```python
from build123d import *

# Parameters (mm, degrees)
SKETCH3_R           = 5.25
SKETCH3_R_2         = 21
BOSS_EXTRUDE1_DEPTH = 2


with BuildPart() as part:
    # Sketch3 → Boss-Extrude1 (new body)
    with BuildSketch(Plane.XY):
        with BuildLine():
            Line((8.459051694, 42.833333333), (25.377155081, 16))
            ThreePointArc((25.377155081, 16), (30, 0), (25.377155081, -16))
            Line((25.377155081, -16), (8.459051694, -42.833333333))
            ThreePointArc((8.459051694, -42.833333333), (0, -47.5), (-8.459051694, -42.833333333))
            Line((-8.459051694, -42.833333333), (-25.377155081, -16))
            ThreePointArc((-25.377155081, -16), (-30, 0), (-25.377155081, 16))
            Line((-25.377155081, 16), (-8.459051694, 42.833333333))
            ThreePointArc((-8.459051694, 42.833333333), (0, 47.5), (8.459051694, 42.833333333))
        make_face()
        with Locations((0, 37.5)):
            Circle(SKETCH3_R, mode=Mode.SUBTRACT)
        Circle(SKETCH3_R_2, mode=Mode.SUBTRACT)
        with Locations(Location((0, -37.5, 0), (0, 0, 180))):
            Circle(SKETCH3_R, mode=Mode.SUBTRACT)
    extrude(amount=BOSS_EXTRUDE1_DEPTH)


solid = part.part
```
Work out the finished part from the listing and answer in its coordinate system (mm). Coordinates: 2 decimals unless noted, no trailing zeros. Order: outer loops, then holes, each group sorted by start corner. A loop starts at its lowest first (then second) coordinate and runs counter-clockwise, first axis right, second up. Notation, with made-up numbers: M 18,-33 L 74,-33 A26 cw 74,-1 Z; hole C 79.5,-20 d4. An arc over 180 degrees is marked long. Use CSV: the item, a comma, the result in double quotes.
1) Section A-A on z = 0.5 is taken. Write down the section's boundary in (x, y), plus the area to 3 significant figures.
Worked out:
outline,"M -25.38,-16 L -8.46,-42.83 A10 ccw 8.46,-42.83 L 25.38,-16 A30 ccw 25.38,16 L 8.46,42.83 A10 ccw -8.46,42.83 L -25.38,16 A30 ccw Z; hole C 0,0 d42; hole C 0,-37.5 d10.5; hole C 0,37.5 d10.5"
area,"2,190 mm^2"
2) Section D-D on x = -14.5 is taken. Write down the section's boundary in (y, z), plus the area to 3 significant figures.
Worked out:
outline,"M -33.25,0 L -15.19,0 L -15.19,2 L -33.25,2 Z; M 15.19,0 L 33.25,0 L 33.25,2 L 15.19,2 Z"
area,"72.2 mm^2"
3) Determine the mould class of faces 1 (the face through (-16.8, -29.604, 0.986)), 2 (the face through (-0.1, 47.5, 1)), 3 (the face through (20.03, 6.31, 0.99)) for opening direction X: released by +X, released by -X, zero draft, split by the parting line, or undercut.
Worked out:
face 1,"released by -X"
face 2,"split by the parting line"
face 3,"undercut"
4) Section B-B on x = 0 is taken. Write down the section's boundary in (y, z).
Worked out:
outline,"M -47.5,0 L -42.75,0 L -42.75,2 L -47.5,2 Z; M -32.25,0 L -21,0 L -21,2 L -32.25,2 Z; M 21,0 L 32.25,0 L 32.25,2 L 21,2 Z; M 42.75,0 L 47.5,0 L 47.5,2 L 42.75,2 Z"
5) Flat-ended cylindrical pins translate along their axes: pin 1 Ø10 at (x, y) = (19.5, 18.5) entering from -Z; pin 2 Ø1 at (x, z) = (22.5, 0.5) entering from +Y. Find the tip coordinate at first contact, or state that the pin passes through.
Worked out:
pin 1,"stops at z = 0"
pin 2,"stops at y = 21.36"
6) Consider line 1 (Y direction, x = 0, z = 1.4); line 2 (Y direction, x = 2, z = 0.6); line 3 (X direction, y = -36, z = 1.7). Determine where each line is inside the solid, lowest interval first. Write a range as [from, to].
Worked out:
line 1,"y = [-47.5, -42.75], [-32.25, -21], [21, 32.25], [42.75, 47.5]"
line 2,"y = [-47.3, -42.35], [-32.65, -20.9], [20.9, 32.65], [42.35, 47.3]"
line 3,"x = [-12.77, -5.03], [5.03, 12.77]"
7) Section C-C on y = 37.5 is taken. Write down the section's boundary in (x, z).
Worked out:
outline,"M -11.82,0 L -5.25,0 L -5.25,2 L -11.82,2 Z; M 5.25,0 L 11.82,0 L 11.82,2 L 5.25,2 Z"
